For this review, use the dimensioned drawing (mm, ordinates from the lowest corner) and the shaded views. A direction names the side the tool comes from. Give positions to 0.01 mm unless a question says otherwise; leave off trailing zeros. Order: outer loops, then holes, each group sorted by start corner. A loop starts at its lowest first (then second) coordinate and runs counter-clockwise, first axis right, second up.
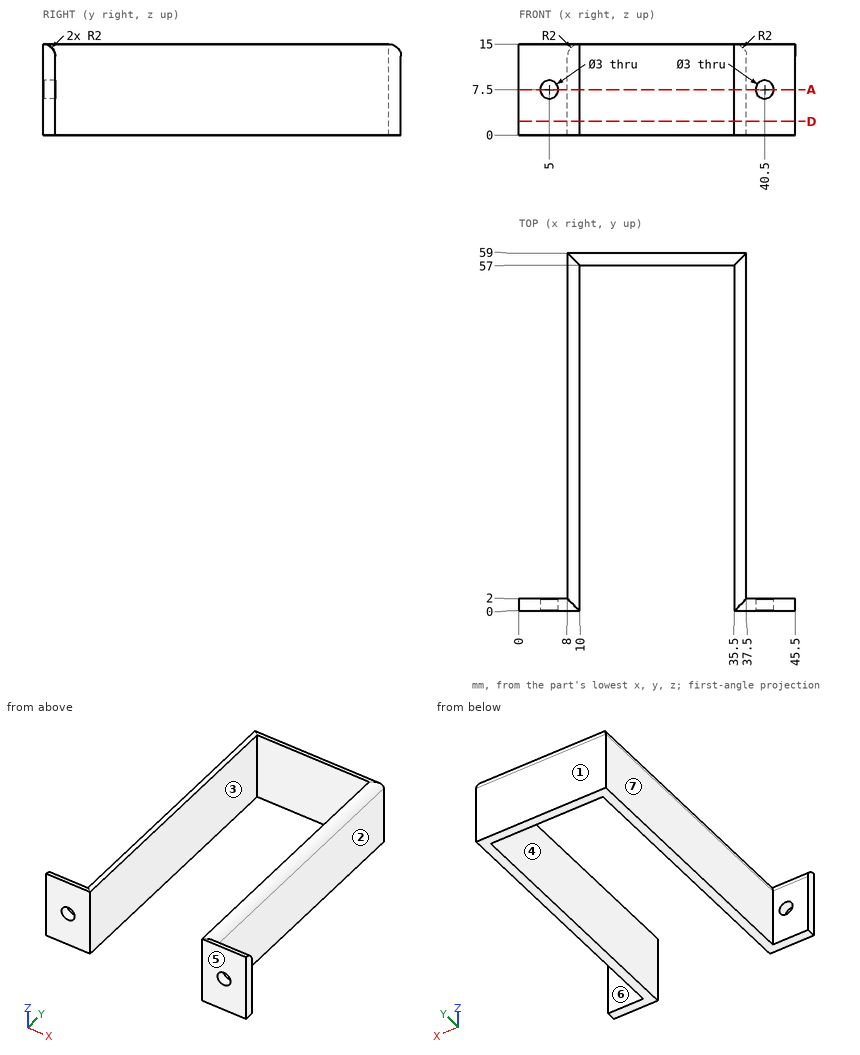
1. Take a section at A-A (z = 7.5). State the section outline as (x, y) points, then the cut area to 3 significant figures.
Recorded:
outline: (0, 0) - (3.5, 0) - (3.5, 2) - (0, 2) - close; (6.5, 0) - (10, 0) - (10, 57) - (35.5, 57) - (35.5, 0) - (39, 0) - (39, 2) - (37.5, 2) - (37.5, 59) - (8, 59) - (8, 2) - (6.5, 2) - close; (42, 0) - (45.5, 0) - (45.5, 2) - (42, 2) - close
area: 307 mm2
2. For line 1 along X through (y, z) = (37, 6.5); line 2 along Y through (x, z) = (18, 8.75); line 3 along Z through (x, y) = (40, 1), list the stretches that pass through material, from the lowest coordinate up.
Recorded:
line 1: x = 8 to 10, 35.5 to 37.5
line 2: y = 57 to 59
line 3: z = 0 to 6.09, 8.91 to 14.73
3. For pin 1 (3 mm diameter, centred on y = 40.5, z = 13, fed in from +X); pin 2 (4 mm diameter, centred on x = 43.5, z = 3.5, fed in from +Y); pin 3 (5 mm diameter, centred on y = 50.5, z = 7.5, fed in from -X); pin 4 (3 mm diameter, centred on x = 33.5, y = 40, fed in from -Z), all flat-tipped, find the tip position at first contact; note any pin that passes through.
Recorded:
pin 1: stops at x = 37.5
pin 2: stops at y = 2
pin 3: stops at x = 8
pin 4: passes through
4. Take a section at D-D (z = 2.25). State the section outline as (x, y) points.
Recorded:
outline: (0, 0) - (10, 0) - (10, 57) - (35.5, 57) - (35.5, 0) - (45.5, 0) - (45.5, 2) - (37.5, 2) - (37.5, 59) - (8, 59) - (8, 2) - (0, 2) - close
5. Draft analysis for pull direction X (two halves, no side actions). For the marked faces 1, 2 and 3, state which applies: pulls with the +X half, pulls with the -X half, needs draft (parallel to the pull), parting line crosses it, or undercut.
Recorded:
face 1: needs draft
face 2: pulls with the +X half
face 3: undercut
6. Machinability: for the marked faces 4, 5, 6 and 7, which of the approach directions +Z, -Z, +X, -X, +Y, -Y give a long, thin tool a straight path to every point of the face, cutting with its end or side? Answer none if there is none.
Recorded:
face 4: +Z, -Z, -Y
face 5: +Z, -Z, +X, -X, -Y
face 6: +Z, -Z, +X, +Y
face 7: +Z, -Z, -X, +Y
